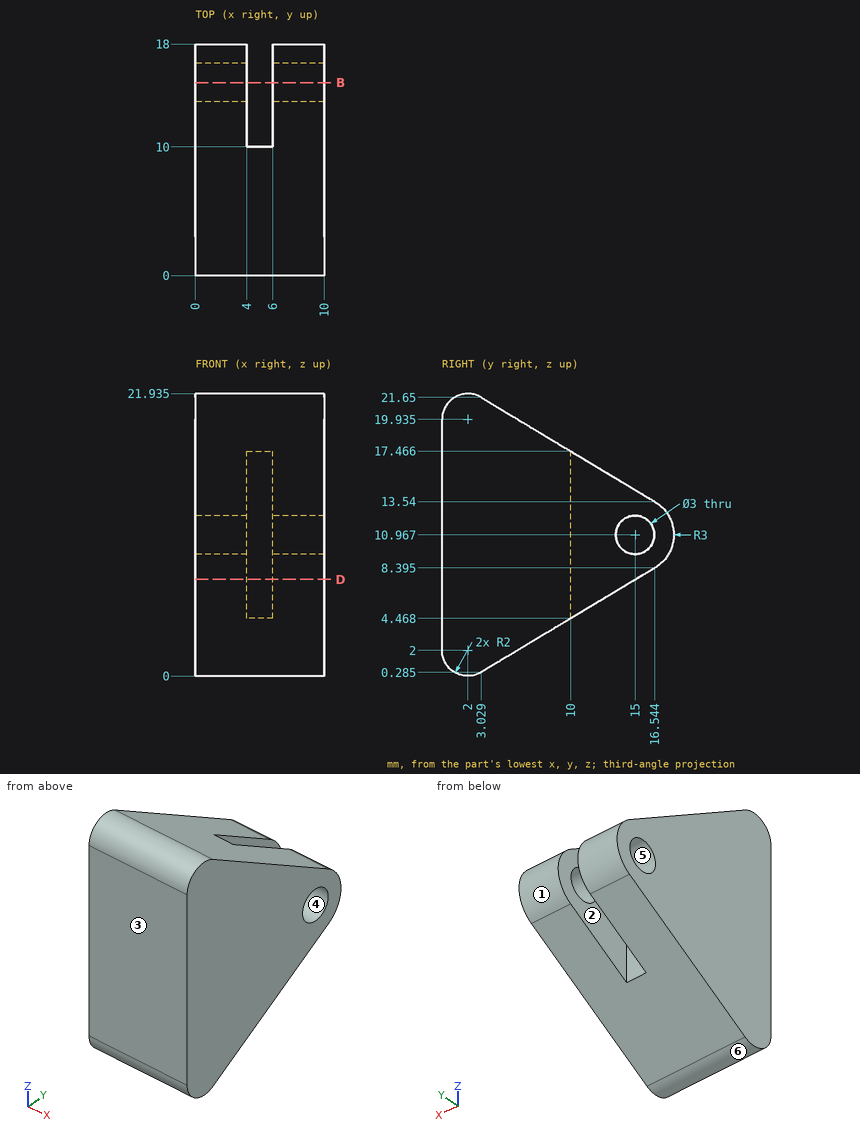
Geometry check sheet. Reference: drawing and pictorial views, mm from the part's lowest x, y, z. A direction names the side the tool comes from. Round coordinates to 2 decimals unless told otherwise and drop trailing zeros. Loops run counter-clockwise (first coordinate to the right, second up) from the corner with the lowest first, then second, coordinate; pieces in that order, holes last. Notation, with made-up numbers: M -21.75,-1.5 L -2.75,-1.5 A36 cw -2.75,36.5 Z; hole C 4.5,10 d11. An arc over 180 degrees is marked long. Return JSON: item names as keys, results as strings. Group by question number.
(1) Section check D-D, the plane z = 7.5. Enter the section's corners in (x, y).
(2) Scan lines: line 1 along X through (y, z) = (14.5, 13.5); line 2 along Y through (x, z) = (4.25, 12.5); line 3 along Y through (x, z) = (1.5, 2) (1 decimal). Record each from-to range of solid material in increasing order. Write a range as [from, to].
(3) Section check B-B, the plane y = 15. Enter the section's corners in (x, z).
(4) Set-up check for the marked faces 1 and 2: record each of +Z, -Z, +X, -X, +Y, -Y from which the full face is reachable in a straight line by a thin tool's end or side.
(5) Go/stop test with flat-tipped pins: pin 1 (4 mm diameter, centred on y = 14.5, z = 9.5, fed in from -X); pin 2 (2.5 mm diameter, centred on y = 15, z = 10.97, fed in from +X); pin 3 (4 mm diameter, centred on x = 3, y = 7, fed in from -Z). Record where each tip stops, or that it passes through.
(6) Mould release check, pull along Y, two halves, no side actions. Record for the marked faces 3, 4, 5 and 6: pulls with the +Y half, pulls with the -Y half, needs draft (parallel to the pull), parting line crosses it, or undercut.
Data:
{
 "1": {"outline": "M 0,0 L 10,0 L 10,15.05 L 6,15.05 L 6,10 L 4,10 L 4,15.05 L 0,15.05 Z"},
 "2": {"line 1": "[0, 4], [6, 10]", "line 2": "[0, 10]", "line 3": "[0, 5.9]"},
 "3": {"outline": "M 0,7.47 L 4,7.47 L 4,9.47 L 0,9.47 Z; M 0,12.47 L 4,12.47 L 4,14.47 L 0,14.47 Z; M 6,7.47 L 10,7.47 L 10,9.47 L 6,9.47 Z; M 6,12.47 L 10,12.47 L 10,14.47 L 6,14.47 Z"},
 "4": {"face 1": "+X, -X, +Y", "face 2": "+Z, -Z, +Y"},
 "5": {"pin 1": "x = 0", "pin 2": "through", "pin 3": "z = 1.47"},
 "6": {"face 3": "pulls with the -Y half", "face 4": "undercut", "face 5": "undercut", "face 6": "parting line crosses it"}
}
